```python
from build123d import *

# Parameters (mm, degrees)
SKETCH_1_W                   = 32
SKETCH_1_H                   = 14
EXTRUDE_1_DEPTH              = 10
SKETCH_2_R                   = 7.6
CUT_EXTRUDE_1_DEPTH          = 2.6
CUT_EXTRUDE_2_DEPTH          = 21.124611797
CUT_EXTRUDE_2_DEPTH_BACK     = 21.124611797
SKETCH_3_R                   = 6.5
SKETCH_4_R                   = 1
CUT_EXTRUDE_3_DEPTH          = 21.124611797
HOLE_WIZARD_M3_1_D           = 3.6
HOLE_WIZARD_M3_1_DEPTH       = 10
HOLE_WIZARD_M3_1_CBORE_D     = 6.5
HOLE_WIZARD_M3_1_CBORE_DEPTH = 3.4


with BuildPart() as part:
    # 草圖1 → 填料-伸長1 (new body)
    with BuildSketch(Plane(origin=(0, 0, 0), x_dir=(1, 0, 0), z_dir=(0, 1, 0))):
        Rectangle(SKETCH_1_W, SKETCH_1_H)
    extrude(amount=EXTRUDE_1_DEPTH)

    # 草圖2 → 除料-伸長1 (cut, symmetric)
    with BuildSketch(Plane.XY):
        with Locations((0, 10)):
            Circle(SKETCH_2_R)
    extrude(amount=CUT_EXTRUDE_1_DEPTH, both=True, mode=Mode.SUBTRACT)

    # 草圖3 → 除料-伸長2 (cut, two sides: drawn at the far end of the back side and taken through both)
    with BuildSketch(Plane.XY.offset(-CUT_EXTRUDE_2_DEPTH_BACK)):
        with Locations((0, 10)):
            Circle(SKETCH_3_R)
    extrude(amount=CUT_EXTRUDE_2_DEPTH + CUT_EXTRUDE_2_DEPTH_BACK, mode=Mode.SUBTRACT)

    # 草圖4 → 除料-伸長3 (cut, through all)
    with BuildSketch(Plane(origin=(0, 10, 0), x_dir=(1, 0, 0), z_dir=(0, 1, 0))):
        with Locations(Location((-12, 0, 0), (0, 0, 270))):
            Circle(SKETCH_4_R)
        with Locations(Location((12, 0, 0), (0, 0, 90))):
            Circle(SKETCH_4_R)
    extrude(amount=-CUT_EXTRUDE_3_DEPTH, mode=Mode.SUBTRACT)

    # M3 六角承窩頭蓋螺釘的柱孔1
    with Locations(Plane(origin=(0, 0, 0), x_dir=(-1, 0, 0), z_dir=(0, -1, 0))):
        with Locations((-12, 0), (12, 0)):
            CounterBoreHole(HOLE_WIZARD_M3_1_D / 2, HOLE_WIZARD_M3_1_CBORE_D / 2, HOLE_WIZARD_M3_1_CBORE_DEPTH, depth=HOLE_WIZARD_M3_1_DEPTH)


solid = part.part
```
Source: CAD feature listing. Evaluate the final solid. Frame: model axes, mm. A direction names the side the tool comes from. Give positions to 0.01 mm unless a question says otherwise; leave off trailing zeros. Loops run counter-clockwise (first coordinate to the right, second up) from the corner with the lowest first, then second, coordinate; pieces in that order, holes last. Notation, with made-up numbers: M 83.25,-24.75 L 139.25,-24.75 A15 ccw 139.25,0.25 Z; hole C -28.75,50.25 d7. An arc over 180 degrees is marked long. Put each result on its own line as item: value.
Q1. Pin query (flat end, axial travel): P1, Ø2.5, axis at x = -2.5, y = 7, coming from the -Z side; P2, Ø4, axis at x = -12, z = 0, coming from the -Y side. Return the tip coordinate at first contact, or that it passes through.
Response values:
P1: passes through
P2: stops at y = 3.4
Q2. Section C-C (z = 0). Return the cut outline in (x, y).
Response values:
outline: M -16,0 L -15.25,0 L -15.25,3.4 L -13.8,3.4 L -13.8,10 L -16,10 Z; M -10.2,3.4 L -8.75,3.4 L -8.75,0 L 8.75,0 L 8.75,3.4 L 10.2,3.4 L 10.2,10 L 7.6,10 A7.6 cw -7.6,10 L -10.2,10 Z; M 13.8,3.4 L 15.25,3.4 L 15.25,0 L 16,0 L 16,10 L 13.8,10 Z
Q3. Line query: probe 1 along Z at (x, y) = (12, 6.5); probe 2 along X at (y, z) = (5, 0.5); probe 3 along X at (y, z) = (4, -0.5). Output: solid intervals per line, ascending. Write a range as [from, to].
Response values:
probe 1: z = [-7, -1.8], [1.8, 7]
probe 2: x = [-16, -13.73], [-10.27, -5.72], [5.72, 10.27], [13.73, 16]
probe 3: x = [-16, -13.73], [-10.27, -4.66], [4.66, 10.27], [13.73, 16]
Q4. Section B-B (y = 6). Return the cut outline in (x, z), and give its area (3 significant figures).
Response values:
outline: M -16,-7 L -5.12,-7 L -5.12,-2.6 L -6.46,-2.6 L -6.46,2.6 L -5.12,2.6 L -5.12,7 L -16,7 Z; M 5.12,-7 L 16,-7 L 16,7 L 5.12,7 L 5.12,2.6 L 6.46,2.6 L 6.46,-2.6 L 5.12,-2.6 Z; hole C -12,0 d3.6; hole C 12,0 d3.6
area: 270 mm²
Q5. Reachability of faces 4 (the cylindrical face through (15.247, 1.676, -0.143)), 5 (the cylindrical face through (-0.17, 2.4, 0.04)), 6 (the flat face through (0, 0, 0)) from +Z, -Z, +X, -X, +Y, -Y: full face, straight path, thin tool, end or side. Return the list, or none.
Response values:
face 4: -Y
face 5: +Y
face 6: +Z, -Z, +X, -X, -Y
Q6. Section D-D (x = 0). Return the cut outline in (y, z).
Response values:
outline: M 0,-7 L 3.5,-7 L 3.5,-2.6 L 2.4,-2.6 L 2.4,2.6 L 3.5,2.6 L 3.5,7 L 0,7 Z
Q7. Section A-A (x = 12). Return the cut outline in (y, z).
Response values:
outline: M 0,-7 L 10,-7 L 10,-1.8 L 3.4,-1.8 L 3.4,-3.25 L 0,-3.25 Z; M 0,3.25 L 3.4,3.25 L 3.4,1.8 L 10,1.8 L 10,7 L 0,7 Z
Q8. Mould query, pull axis Z, two halves, no side actions, for faces 1 (the cylindrical face through (10.2, 6.75, -0.08)), 2 (the flat face through (-10, 10, -2)), 3 (the flat face through (0, 3, 7)). Classes: released by +Z, released by -Z, zero draft, split by the parting line, or undercut.
Response values:
face 1: undercut
face 2: zero draft
face 3: released by +Z
